Here's how the part is built. I have some questions about the finished solid (model axes, mm). Coordinates: 2 decimals unless noted, no trailing zeros. Order: outer loops, then holes, each group sorted by start corner. A loop starts at its lowest first (then second) coordinate and runs counter-clockwise, first axis right, second up. Notation, with made-up numbers: (61.25, 7) - (94.25, 7) arc R13 ccw to (94.25, 20) - close; hole circle Ø9 at (-38, -34). An arc over 180 degrees is marked (long way). Answer as CSV lines item,"result". Start each with the question number.
Q1. I need wall thicknesses on line 1 (Z direction, x = 3.5, y = -8); line 2 (Y direction, x = 3.5, z = 24); line 3 (Z direction, x = 5.75, y = -3). Which ranges of each line are inside material? Lowest first, please.
Q2. For pin 1 Ø1.5 at (x, z) = (6, 6.5) entering from -Y; pin 2 Ø4 at (x, z) = (4.5, 17) entering from -Y, each with a flat end and sliding along its axis, tell me the tip position at first contact or that it passes through.
Q3. Suppose I cut it at C-C (z = 3). Please give me the cut outline in (x, y), then the cut area to 3 significant figures.
Q4. Suppose I cut it at A-A (y = -0.25). Please give me the cut outline in (x, z), then the cut area to 3 significant figures.
Q5. Thinking about a two-plate mould opening in Z: for faces 1 (the face through (3, -3, 0)), 2 (the face through (3, -3, 30)), 3 (the face through (6.935, -2.818, 5.149)), which applies, released by +Z, released by -Z, zero draft, split by the parting line, or undercut?
Q6. Suppose I cut it at B-B (x = 3). Please give me the cut outline in (y, z).
Q7. Suppose I cut it at D-D (y = 1.5). Please give me the cut outline in (x, z), then the cut area to 3 significant figures.
from build123d import *

# Parameters (mm, degrees)
F0_W     = 20
F0_H     = 20
F1_DEPTH = 30
F3_R     = 3.4
F4_DEPTH = 25
F2_R     = 3.4
F5_DEPTH = 25
F6_W     = 20
F6_H     = 20
F6_R     = 6.5
F7_DEPTH = 30


with BuildPart() as f1:
    # F0 (on Top) → F1 (new body)
    with BuildSketch(Plane.XY):
        with Locations((3.538307, -2.90917)):
            Rectangle(F0_W, F0_H)
    extrude(amount=F1_DEPTH)

    # F3 (on face) → F4 (cut)
    with BuildSketch(Plane.YZ.offset(13.538307)):
        with Locations((-2.90917, 24)):
            Circle(F3_R)
    extrude(amount=-F4_DEPTH, mode=Mode.SUBTRACT)

    # F2 (on face) → F5 (cut)
    with BuildSketch(Plane(origin=(0, 7.09083, 0), x_dir=(-1, 0, 0), z_dir=(0, 1, 0))):
        with Locations((-3.538307, 5)):
            Circle(F2_R)
    extrude(amount=-F5_DEPTH, mode=Mode.SUBTRACT)

    # F6 (on face) → F7 (cut)
    with BuildSketch(Plane(origin=(0, 0, 0), x_dir=(1, 0, 0), z_dir=(0, 0, -1))):
        with Locations((3.538307, 2.90917)):
            Rectangle(F6_W, F6_H)
        with Locations((3.538307, 2.90917)):
            Circle(F6_R, mode=Mode.SUBTRACT)
    extrude(amount=-F7_DEPTH, mode=Mode.SUBTRACT)


solid = f1.part
Here are the results:
1,line 1,"z = 0 to 1.6, 8.4 to 30"
1,line 2,"y = -9.41 to -6.31, 0.49 to 3.59"
1,line 3,"z = 0 to 2.42, 7.58 to 20.6, 27.4 to 30"
2,pin 1,"stops at y = -8.89"
2,pin 2,"stops at y = -9.41"
3,outline,"(0.79, -8.8) - (0.79, 2.98) arc R6.5 ccw to start; (6.29, -8.8) arc R6.5 ccw to (6.29, 2.98) - close"
3,area,"63.4 mm²"
4,outline,"(-2.39, 0) - (9.47, 0) - (9.47, 21.88) - (-2.39, 21.88) - close; (-2.39, 26.12) - (9.47, 26.12) - (9.47, 30) - (-2.39, 30) - close; hole circle Ø6.8 at (3.54, 5)"
4,area,"269 mm²"
5,face 1,"released by -Z"
5,face 2,"released by +Z"
5,face 3,"undercut"
6,outline,"(-9.39, 0) - (3.57, 0) - (3.57, 1.64) - (-9.39, 1.64) - close; (-9.39, 8.36) - (3.57, 8.36) - (3.57, 30) - (-9.39, 30) - close; hole circle Ø6.8 at (-2.91, 24)"
7,outline,"(-1.24, 0) - (8.31, 0) - (8.31, 30) - (-1.24, 30) - close; hole circle Ø6.8 at (3.54, 5)"
7,area,"250 mm²"
